Geometry check sheet. Reference: drawing and pictorial views, mm from the part's lowest x, y, z. Round coordinates to 2 decimals unless told otherwise and drop trailing zeros. Write each loop counter-clockwise with the first axis right and the second up, starting at its lowest first coordinate (ties: lowest second). Pieces come first, ordered by that corner, then holes. Notation, with made-up numbers: (49.25, -8.5) -> (62.25, -8.5) arc R36 ccw to (62.25, 27.5) -> close; hole circle Ø1 at (41.25, -25). An arc over 180 degrees is marked (long way). Answer as a JSON object with one key per item and string values. Group by question number.
(1) Sectioned sample at D-D on x = 1.15. Record the cut outline in (y, z) (3 decimals), and give its area (3 significant figures).
(2) Gauge pin test, flat end, axial feed: pin 1 Ø1.5 at (x, y) = (3, 8.5) entering from +Z. Record the tip position at first contact, or that the pin passes through.
(3) Sectioned sample at C-C on y = 15.5. Record the cut outline in (x, z), and give its area (3 significant figures).
(4) Sectioned sample at B-B on x = 2. Record the cut outline in (y, z) (3 decimals).
(5) Draft check along Y on the marked faces 1, 2, 3 and 4. Enter one of: released by +Y, released by -Y, zero draft, split by the parting line, or undercut.
(6) Scan lines: L1, parallel to Y at x = 2.55, z = 6.35 (3 decimals); L2, parallel to Y at x = 2.8, z = 6.35 (3 decimals); L3, parallel to Y at x = 0.5, z = 6.5. Record each from-to range of solid material in increasing order. Write a range as from..to.
(7) Sectioned sample at A-A on z = 6.35. Record the cut outline in (x, y) (3 decimals), and give its area (3 significant figures).
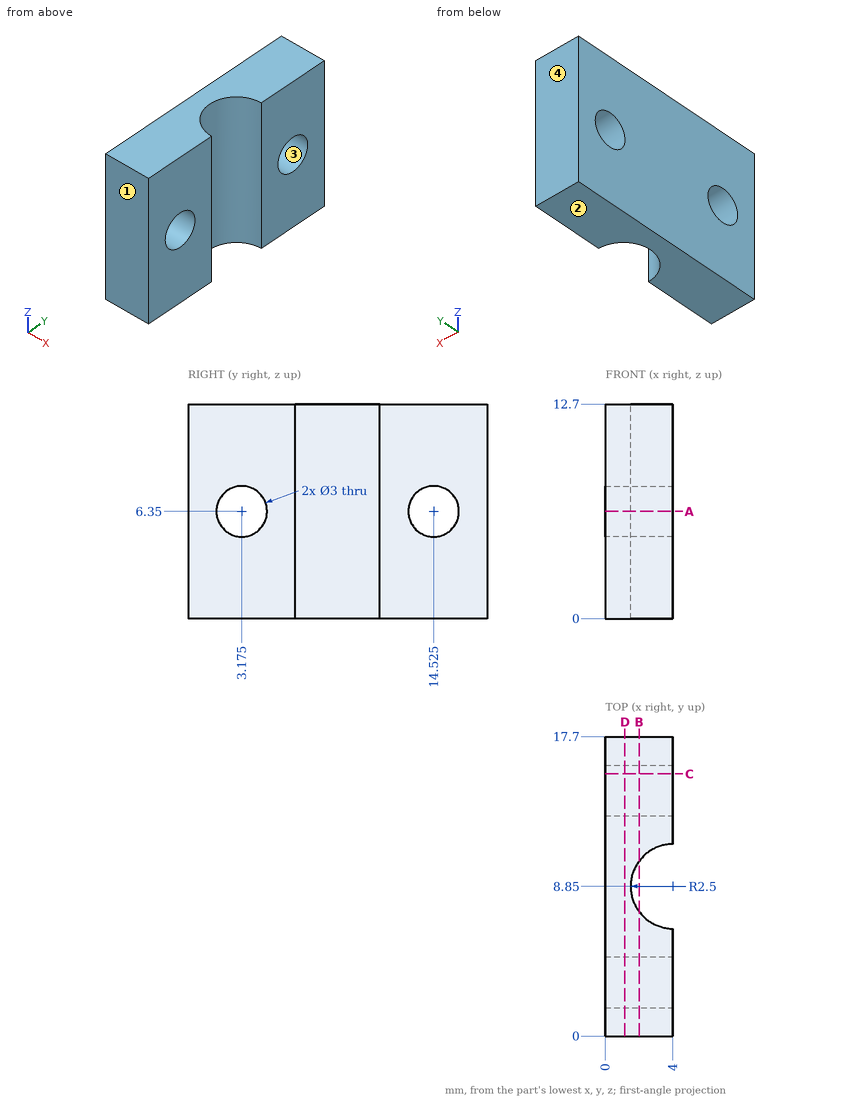
Computed values:
{
 "1": {"outline": "(0, 0) -> (17.7, 0) -> (17.7, 12.7) -> (0, 12.7) -> close; hole circle Ø3 at (3.175, 6.35); hole circle Ø3 at (14.525, 6.35)", "area": "211 mm2"},
 "2": {"pin 1": "through"},
 "3": {"outline": "(0, 0) -> (4, 0) -> (4, 5.21) -> (0, 5.21) -> close; (0, 7.49) -> (4, 7.49) -> (4, 12.7) -> (0, 12.7) -> close", "area": "41.7 mm2"},
 "4": {"outline": "(0, 0) -> (7.35, 0) -> (7.35, 12.7) -> (0, 12.7) -> close; (10.35, 0) -> (17.7, 0) -> (17.7, 12.7) -> (10.35, 12.7) -> close; hole circle Ø3 at (3.175, 6.35); hole circle Ø3 at (14.525, 6.35)"},
 "5": {"face 1": "released by -Y", "face 2": "zero draft", "face 3": "undercut", "face 4": "released by +Y"},
 "6": {"L1": "0..1.675, 4.675..6.813, 10.887..13.025, 16.025..17.7", "L2": "0..1.675, 4.675..6.657, 11.043..13.025, 16.025..17.7", "L3": "0..1.68, 4.67..13.03, 16.02..17.7"},
 "7": {"outline": "(0, 0) -> (4, 0) -> (4, 1.675) -> (0, 1.675) -> close; (0, 4.675) -> (4, 4.675) -> (4, 6.35) arc R2.5 cw to (4, 11.35) -> (4, 13.025) -> (0, 13.025) -> close; (0, 16.025) -> (4, 16.025) -> (4, 17.7) -> (0, 17.7) -> close", "area": "37.0 mm2"}
}
